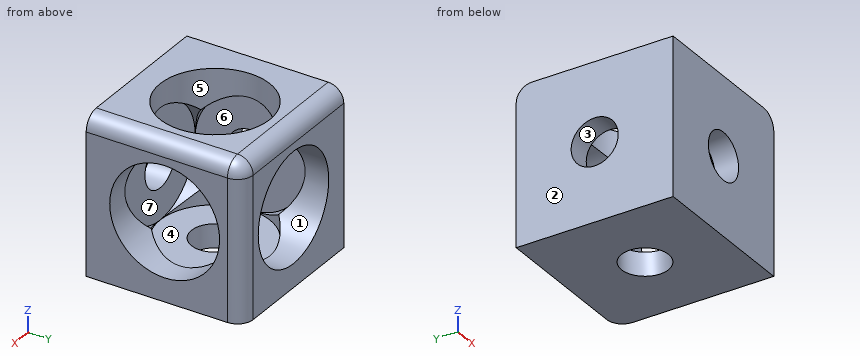
from build123d import *

# Parameters (mm, degrees)
ESQUISSE1_W             = 20
ESQUISSE1_H             = 20
BOSS_EXTRU_1_DEPTH      = 20
CONG_1_R                = 2
ESQUISSE2_R             = 3
ENL_V_MAT_EXTRU_1_DEPTH = 21
ESQUISSE3_R             = 3
ENL_V_MAT_EXTRU_2_DEPTH = 21
ESQUISSE4_R             = 3
ENL_V_MAT_EXTRU_3_DEPTH = 21
ESQUISSE5_R             = 7
ENL_V_MAT_EXTRU_4_DEPTH = 17
ESQUISSE6_R             = 7
ENL_V_MAT_EXTRU_5_DEPTH = 17
ESQUISSE7_R             = 7
ENL_V_MAT_EXTRU_6_DEPTH = 17


with BuildPart() as part:
    # Esquisse1 → Boss.-Extru.1 (new body)
    with BuildSketch(Plane.XY):
        with Locations((-10, 10)):
            Rectangle(ESQUISSE1_W, ESQUISSE1_H)
    extrude(amount=BOSS_EXTRU_1_DEPTH)

    # Congé1
    cong_1_edges = [part.edges().sort_by_distance(p)[0] for p in [
        (0, 10, 20),
        (-10, 20, 20),
        (0, 20, 10),
    ]]
    fillet(cong_1_edges, radius=CONG_1_R)

    # Esquisse2 → Enlèv. mat.-Extru.1 (cut, through all)
    with BuildSketch(Plane.XY.offset(20)):
        with Locations((-10, 10)):
            Circle(ESQUISSE2_R)
    extrude(amount=-ENL_V_MAT_EXTRU_1_DEPTH, mode=Mode.SUBTRACT)

    # Esquisse3 → Enlèv. mat.-Extru.2 (cut, through all)
    with BuildSketch(Plane(origin=(0, 0, 0), x_dir=(0, 0, -1), z_dir=(1, 0, 0))):
        with Locations(Location((-10, 10, 0), (0, 0, 90))):  # turned: the seam where the file's is
            Circle(ESQUISSE3_R)
    extrude(amount=-ENL_V_MAT_EXTRU_2_DEPTH, mode=Mode.SUBTRACT)

    # Esquisse4 → Enlèv. mat.-Extru.3 (cut, through all)
    with BuildSketch(Plane(origin=(0, 20, 0), x_dir=(-1, 0, 0), z_dir=(0, 1, 0))):
        with Locations(Location((10, 10, 0), (0, 0, 90))):  # turned: the seam where the file's is
            Circle(ESQUISSE4_R)
    extrude(amount=-ENL_V_MAT_EXTRU_3_DEPTH, mode=Mode.SUBTRACT)

    # Esquisse5 → Enlèv. mat.-Extru.4 (cut)
    with BuildSketch(Plane.XY.offset(20)):
        with Locations((-10, 10)):
            Circle(ESQUISSE5_R)
    extrude(amount=-ENL_V_MAT_EXTRU_4_DEPTH, mode=Mode.SUBTRACT)

    # Esquisse6 → Enlèv. mat.-Extru.5 (cut)
    with BuildSketch(Plane(origin=(0, 0, 0), x_dir=(0, 0, -1), z_dir=(1, 0, 0))):
        with Locations(Location((-10, 10, 0), (0, 0, 90))):  # turned: the seam where the file's is
            Circle(ESQUISSE6_R)
    extrude(amount=-ENL_V_MAT_EXTRU_5_DEPTH, mode=Mode.SUBTRACT)

    # Esquisse7 → Enlèv. mat.-Extru.6 (cut)
    with BuildSketch(Plane(origin=(0, 20, 0), x_dir=(1, 0, 0), z_dir=(0, 1, 0))):
        with Locations(Location((-10, -10, 0), (0, 0, 270))):  # turned: the seam where the file's is
            Circle(ESQUISSE7_R)
    extrude(amount=-ENL_V_MAT_EXTRU_6_DEPTH, mode=Mode.SUBTRACT)


solid = part.part
Source: CAD feature listing. Evaluate the final solid. Frame: model axes, mm. Face numbers are marked on the shaded views. A direction names the side the tool comes from. Round coordinates to 2 decimals unless told otherwise and drop trailing zeros. Write each loop counter-clockwise with the first axis right and the second up, starting at its lowest first coordinate (ties: lowest second). Pieces come first, ordered by that corner, then holes. Notation, with made-up numbers: (0, -3) - (35, -3) arc R25 ccw to (35, 15) - close; hole circle Ø9 at (49.25, 69.5). An arc over 180 degrees is marked (long way). Use CSV: the item, a comma, the result in double quotes. Start each with the question number.
(1) Material intervals for probe 1 along Y at (x, z) = (-10, 17.1); probe 2 along X at (y, z) = (1.8, 10); probe 3 along Z at (x, y) = (-19, 10), sorted ascending. Write a range as [from, to].
(2) Cut plane C-C, the plane x = -11. Return loops of the section in (y, z).
(3) Set-up query: the marked faces 5, 6 and 7. Return all of +Z, -Z, +X, -X, +Y, -Y with unobstructed straight access to the full face (end or side cutting, diameter ignored); none if empty.
(4) First-contact query: pin 1 Ø5 at (x, y) = (-9, 7.5) entering from +Z; pin 2 Ø11 at (y, z) = (8, 13.5) entering from +X; pin 3 Ø11 at (y, z) = (10, 10) entering from +X; pin 4 Ø7 at (x, z) = (-12, 9.5) entering from +Y. Flat tips, straight axial feed; report the tip coordinate or a pass-through.
(5) Cut plane A-A, the plane x = -4.75. Return loops of the section in (y, z).
(6) Mould query, pull axis Z, two halves, no side actions, for the marked faces 1, 2, 3 and 4. Classes: pulls with the +Z half, pulls with the -Z half, needs draft (parallel to the pull), parting line crosses it, or undercut.
(7) Cut plane D-D, the plane z = 2. Return loops of the section in (x, y).
(8) Cut plane B-B, the plane z = 10.5. Give the number of separate pieces and of enclosed holes in the cut face, and give its area (3 significant figures).
Geometry says:
1,probe 1,"[0, 3], [17, 20]"
1,probe 2,"[-20, -13], [-7, 0]"
1,probe 3,"[0, 7], [13, 20]"
2,outline,"(0, 0) - (7.17, 0) - (7.17, 3) - (3.07, 3) - (3.07, 3.07) - (3, 3.07) - (3, 7.17) - (0, 7.17) - close; (0, 12.83) - (3, 12.83) - (3, 16.93) - (3.07, 16.93) - (3.07, 20) - (0, 20) - close; (12.83, 0) - (20, 0) - (20, 3.07) - (16.93, 3.07) - (16.93, 3) - (12.83, 3) - close; (16.93, 16.93) - (20, 16.93) - (20, 18) arc R2 ccw to (18, 20) - (16.93, 20) - close"
3,face 5,"+Z"
3,face 6,"+X"
3,face 7,"+Y"
4,pin 1,"z = 3"
4,pin 2,"x = 0"
4,pin 3,"x = -17"
4,pin 4,"y = 3"
5,outline,"(0, 0) - (20, 0) - (20, 5.37) - (15.25, 5.37) arc R7 cw to (14.63, 4.75) - (14.63, 3) - (5.37, 3) - (5.37, 4.75) arc R7 cw to (4.75, 5.37) - (3, 5.37) - (3, 14.63) - (4.75, 14.63) arc R7 cw to (5.37, 15.25) - (5.37, 20) - (0, 20) - close; (14.63, 15.25) arc R7 cw to (15.25, 14.63) - (20, 14.63) - (20, 18) arc R2 ccw to (18, 20) - (14.63, 20) - close"
6,face 1,"undercut"
6,face 2,"needs draft"
6,face 3,"undercut"
6,face 4,"pulls with the +Z half"
7,outline,"(-20, 0) - (0, 0) - (0, 18) arc R2 ccw to (-2, 20) - (-20, 20) - close; hole circle Ø6 at (-10, 10)"
8,separate pieces,"4"
8,enclosed holes,"0"
8,area,"83.9 mm²"
